from build123d import *

# Parameters (mm, degrees)
F0_W     = 40
F0_H     = 40
F1_DEPTH = 3
F2_R     = 4.9
F2_R_2   = 3
F3_DEPTH = 5
F4_R     = 19
F5_DEPTH = 1


with BuildPart() as f1:
    # F0 (on Front) → F1 (new body)
    with BuildSketch(Plane.XZ):
        Rectangle(F0_W, F0_H)
    extrude(amount=F1_DEPTH)

    # F2 (on face) → F3 (join)
    with BuildSketch(Plane(origin=(0, 0, 0), x_dir=(-1, 0, 0), z_dir=(0, 1, 0))):
        Circle(F2_R)
        Circle(F2_R_2, mode=Mode.SUBTRACT)
    extrude(amount=F3_DEPTH)

    # F4 (on face) → F5 (cut)
    with BuildSketch(Plane.XZ.offset(3)):
        Circle(F4_R)
        with BuildLine():
            ThreePointArc((-12.505157, 8.283783), (-12.727922, 12.727922), (-8.283783, 12.505157))
            Line((-8.283783, 12.505157), (1.051123, 3.170251))
            Line((1.051123, 3.170251), (10.559486, 12.678614))
            ThreePointArc((10.559486, 12.678614), (12.727922, 12.727922), (12.678614, 10.559486))
            Line((12.678614, 10.559486), (3.170251, 1.051123))
            Line((3.170251, 1.051123), (12.505157, -8.283783))
            ThreePointArc((12.505157, -8.283783), (12.727922, -12.727922), (8.283783, -12.505157))
            Line((8.283783, -12.505157), (-1.051123, -3.170251))
            Line((-1.051123, -3.170251), (-10.559486, -12.678614))
            ThreePointArc((-10.559486, -12.678614), (-12.727922, -12.727922), (-12.678614, -10.559486))
            Line((-12.678614, -10.559486), (-3.170251, -1.051123))
            Line((-3.170251, -1.051123), (-12.505157, 8.283783))
        make_face(mode=Mode.SUBTRACT)
    extrude(amount=-F5_DEPTH, mode=Mode.SUBTRACT)


solid = f1.part
Design review of the part built by this model. Coordinates are the model's own, in mm. A direction names the side the tool comes from. Coordinates: 2 decimals unless noted, no trailing zeros. Order: outer loops, then holes, each group sorted by start corner. A loop starts at its lowest first (then second) coordinate and runs counter-clockwise, first axis right, second up. Notation, with made-up numbers: (-28, 87) - (14, 87) arc R24 ccw to (14, 102) - close; hole circle Ø7 at (64, 37). An arc over 180 degrees is marked (long way). Put each result on its own line as item: value.
1) The part is to be moulded in two halves that separate along Z. For faces 4 (the face through (0.1, 5, -3.2)), 5 (the face through (1.062, 2.465, -4.783)), 6 (the face through (-7.99, -2.51, -5.87)), say which applies: released by +Z, released by -Z, zero draft, split by the parting line, or undercut.
Response values:
face 4: zero draft
face 5: split by the parting line
face 6: undercut
2) Take a section at B-B, the plane z = 0. Give the boundary of the cut face in (x, y), and give its area (3 significant figures).
Response values:
outline: (-20, -3) - (-19, -3) - (-19, -2) - (-4.22, -2) - (-4.22, -3) - (4.22, -3) - (4.22, -2) - (19, -2) - (19, -3) - (20, -3) - (20, 0) - (4.9, 0) - (4.9, 5) - (3, 5) - (3, 0) - (-3, 0) - (-3, 5) - (-4.9, 5) - (-4.9, 0) - (-20, 0) - close
area: 109 mm²
3) Insertion check: P1, Ø2, axis at x = -0.5, z = 11, coming from the +Y side; P2, Ø4, axis at y = 4, z = -7.5, coming from the -X side. Each pin has a flat end and moves straight along its axis. Give the tip position at first contact, or say it passes through.
Response values:
P1: stops at y = 0
P2: passes through
4) Tool access review of faces 1 (the face through (3, 2, 0)), 2 (the face through (-5.74, -2.51, -7.86)), 3 (the face through (0, -1, 20)): name each direction out of +Z, -Z, +X, -X, +Y, -Y from which nothing blocks a thin tool from reaching the whole face with its end or side.
Response values:
face 1: +Y
face 2: -Y
face 3: +Z, +X, -X, +Y, -Y
5) Take a section at D-D, the plane x = -9. Give the boundary of the cut face in (y, z), and give its area (3 significant figures).
Response values:
outline: (-3, -20) - (0, -20) - (0, 20) - (-3, 20) - (-3, 16.73) - (-2, 16.73) - (-2, 13.14) - (-3, 13.14) - (-3, 4.78) - (-2, 4.78) - (-2, -6.88) - (-3, -6.88) - (-3, -11.12) - (-2, -11.12) - (-2, -16.73) - (-3, -16.73) - close
area: 99.1 mm²
6) Take a section at C-C, the plane y = 2. Give the boundary of the cut face in (x, z).
Response values:
outline: circle Ø9.8 at (0, 0); hole circle Ø6 at (0, 0)
7) Take a section at A-A, the plane x = 6. Give the boundary of the cut face in (y, z), and give its area (3 significant figures).
Response values:
outline: (-3, -20) - (0, -20) - (0, 20) - (-3, 20) - (-3, 18.03) - (-2, 18.03) - (-2, 8.12) - (-3, 8.12) - (-3, 3.88) - (-2, 3.88) - (-2, -1.78) - (-3, -1.78) - (-3, -10.22) - (-2, -10.22) - (-2, -18.03) - (-3, -18.03) - close
area: 96.6 mm²
8) Wall thickness on L1, parallel to Z at x = 0, y = 1.15; L2, parallel to Z at x = 0, y = -2.3; L3, parallel to Z at x = -9, y = -2.25: over which ranges is each line inside the solid? List them lowest first. Write a range as from..to.
Response values:
L1: z = -4.9..-3, 3..4.9
L2: z = -20..-19, -4.22..4.22, 19..20
L3: z = -20..-16.73, -11.12..-6.88, 4.78..13.14, 16.73..20
